from build123d import *

# Parameters (mm, degrees)
CORTE_EXTRUS_O1_DEPTH      = 88.705522097
CORTE_EXTRUS_O1_DEPTH_BACK = 88.705522097
ESBO_O2_W                  = 3.414213562
ESBO_O2_H                  = 19
ESBO_O2_W_2                = 2.65
CORTE_EXTRUS_O2_DEPTH      = 89.018596472
CORTE_EXTRUS_O2_DEPTH_BACK = 89.018596472
ESBO_O3_R                  = 4


with BuildPart() as part:
    # Esboço1 → Revolução1 (revolve)
    with BuildSketch(Plane(origin=(0, 0, 0), x_dir=(0, 0, -1), z_dir=(1, 0, 0)), mode=Mode.PRIVATE) as revolu_o1_sk:
        with BuildLine():
            Line((0, 0), (0, 6))
            Line((0, 6), (0.707106781, 6.707106781))
            Line((0.707106781, 6.707106781), (3.808899287, 6.707106781))
            ThreePointArc((3.808899287, 6.707106781), (6, 4.516006068), (8.191100713, 6.707106781))
            Line((8.191100713, 6.707106781), (87.191100713, 6.707106781))
            Line((87.191100713, 6.707106781), (87.191100713, 0))
            Line((87.191100713, 0), (0, 0))
        make_face()
    revolve(revolu_o1_sk.sketch.rotate(Axis((0, 0, 0), (0, 0, -1)), 90), axis=Axis((0, 0, 0), (0, 0, -1)))

    # Esboço2 → Corte-extrusão1 (cut, two sides: drawn at the far end of the back side and taken through both)
    with BuildSketch(Plane(origin=(0, 0, 0), x_dir=(1, 0, 0), z_dir=(0, 1, 0)).offset(-CORTE_EXTRUS_O1_DEPTH_BACK)):
        with Locations((5, 77.691100713)):
            Rectangle(ESBO_O2_W, ESBO_O2_H)
        with Locations((-5.382106781, 77.691100713)):
            Rectangle(ESBO_O2_W_2, ESBO_O2_H)
    extrude(amount=CORTE_EXTRUS_O1_DEPTH + CORTE_EXTRUS_O1_DEPTH_BACK, mode=Mode.SUBTRACT)

    # Esboço3 → Corte-extrusão2 (cut, two sides: drawn at the far end of the back side and taken through both)
    with BuildSketch(Plane(origin=(3.292893219, 0, 0), x_dir=(0, 0, -1), z_dir=(1, 0, 0)).offset(-CORTE_EXTRUS_O2_DEPTH_BACK)):
        with Locations((79.191100713, 0)):
            Circle(ESBO_O3_R)
    extrude(amount=CORTE_EXTRUS_O2_DEPTH + CORTE_EXTRUS_O2_DEPTH_BACK, mode=Mode.SUBTRACT)


solid = part.part
Read the model definition and answer for the solid it produces. Units are mm, in the model's axes. A direction names the side the tool comes from. Give positions to 0.01 mm unless a question says otherwise; leave off trailing zeros. Write each loop counter-clockwise with the first axis right and the second up, starting at its lowest first coordinate (ties: lowest second). Pieces come first, ordered by that corner, then holes. Notation, with made-up numbers: (71.5, -2.75) - (76.5, -2.75) arc R18 ccw to (76.5, 29.25) - close; hole circle Ø2 at (21.25, 74). An arc over 180 degrees is marked (long way). Use CSV: the item, a comma, the result in double quotes. Start each with the question number.
Item 1: Consider line 1 (Z direction, x = 2, y = 0); line 2 (Z direction, x = 4.5, y = -1.5); line 3 (Y direction, x = 3, z = -20). Determine where each line is inside the solid, lowest interval first.
Item 2: Flat-ended cylindrical pins translate along their axes: P1, Ø1.3, axis at x = -5, y = -2, coming from the -Z side; P2, Ø5, axis at x = 3.5, z = -17, coming from the +Y side; P3, Ø5, axis at x = -4.5, z = -42, coming from the +Y side. Find the tip coordinate at first contact, or state that the pin passes through.
Item 3: The part is cut by section B-B, the plane y = 0. Give the vertices of the cut face in (x, z), and give its area (3 significant figures).
Item 4: The part is cut by section A-A, the plane x = 0. Give the vertices of the cut face in (y, z).
Item 5: For faces 5 (the flat face through (-5, 0, -68.191)), 6 (the cylindrical face through (3, 6, -39)), 7 (the flat face through (3.293, -3, -75)), determine the directions among +Z, -Z, +X, -X, +Y, -Y from which every point of the face is accessible in a straight line to the end or side of a thin tool.
Item 6: The part is cut by section C-C, the plane z = -52. Give the vertices of the cut face in (x, y).
Item 7: The mould has two halves that part along Z. Classify faces 1 (the flat face through (-4.057, 2, -75)), 2 (the flat face through (0, 0, 0)), 3 (the cylindrical face through (-0.434, 0.176, -75.195)), 4 (the flat face through (0, 0, -87.191)): pulls with the +Z half, pulls with the -Z half, needs draft (parallel to the pull), parting line crosses it, or undercut.
Taken from the geometry:
1,line 1,"-87.19 to -83.19, -75.19 to 0"
1,line 2,"-68.19 to -6.97, -5.03 to 0"
1,line 3,"-6 to 6"
2,P1,"z = -68.19"
2,P2,"y = 6.63"
2,P3,"y = 6.4"
3,outline,"(-6.71, -68.19) - (-4.06, -68.19) - (-4.06, -75.19) - (3.29, -75.19) - (3.29, -68.19) - (6.71, -68.19) - (6.71, -8.19) arc R2.19 cw to (6.71, -3.81) - (6.71, -0.71) - (6, 0) - (-6, 0) - (-6.71, -0.71) - (-6.71, -3.81) arc R2.19 cw to (-6.71, -8.19) - close; (-4.06, -87.19) - (3.29, -87.19) - (3.29, -83.19) - (-4.06, -83.19) - close"
3,area,"980 mm2"
4,outline,"(-6.71, -87.19) - (6.71, -87.19) - (6.71, -8.19) arc R2.19 cw to (6.71, -3.81) - (6.71, -0.71) - (6, 0) - (-6, 0) - (-6.71, -0.71) - (-6.71, -3.81) arc R2.19 cw to (-6.71, -8.19) - close; hole circle Ø8 at (0, -79.19)"
5,face 5,"-Z, -X, +Y, -Y"
5,face 6,"+Z, -Z"
5,face 7,"-Z, +X, +Y, -Y"
6,outline,"circle Ø13.41 at (0, 0)"
7,face 1,"needs draft"
7,face 2,"pulls with the +Z half"
7,face 3,"undercut"
7,face 4,"pulls with the -Z half"
